Source: CAD feature listing. Evaluate the final solid. Frame: model axes, mm. A direction names the side the tool comes from. Give positions to 0.01 mm unless a question says otherwise; leave off trailing zeros. Order: outer loops, then holes, each group sorted by start corner. A loop starts at its lowest first (then second) coordinate and runs counter-clockwise, first axis right, second up.
```python
from build123d import *

# Parameters (mm, degrees)
EXTRUDE1_DEPTH           = 311.15
SKETCH2_R                = 5.207
SKETCH2_R_2              = 3.556
SKETCH2_R_3              = 6.731
CUT_WEB_HOLES_DEPTH      = 329.182750394
SKETCH3_R                = 6.731
SKETCH3_R_2              = 5.207
CUT_FLG_HOLES_DEPTH      = 329.182750394
CUT_FLG_HOLES_DEPTH_BACK = 329.182750394
SKETCH6_R                = 5.207
VLV_MODULATOR_DEPTH      = 329.182750394


with BuildPart() as part:
    # Sketch1 → Extrude1 (new, symmetric)
    with BuildSketch(Plane(origin=(0, 0, 0), x_dir=(0, 0, -1), z_dir=(1, 0, 0))):
        with BuildLine():
            Line((57.15, 87.3125), (12.7, 87.3125))
            ThreePointArc((12.7, 87.3125), (3.719743879, 83.592756121), (0, 74.6125))
            Line((0, 74.6125), (0, -74.6125))
            ThreePointArc((0, -74.6125), (3.719743879, -83.592756121), (12.7, -87.3125))
            Line((12.7, -87.3125), (57.15, -87.3125))
            Line((57.15, -87.3125), (57.15, -80.9625))
            Line((57.15, -80.9625), (12.7, -80.9625))
            ThreePointArc((12.7, -80.9625), (8.209871939, -79.102628061), (6.35, -74.6125))
            Line((6.35, -74.6125), (6.35, 74.6125))
            ThreePointArc((6.35, 74.6125), (8.209871939, 79.102628061), (12.7, 80.9625))
            Line((12.7, 80.9625), (57.15, 80.9625))
            Line((57.15, 80.9625), (57.15, 87.3125))
        make_face()
    extrude(amount=EXTRUDE1_DEPTH, both=True)

    # Sketch2 → Cut-Web Holes (cut, through all)
    with BuildSketch(Plane.XY):
        with Locations((-185.7375, 52.3875)):
            Circle(SKETCH2_R)
        with Locations((-261.9375, -4.7625)):
            Circle(SKETCH2_R_2)
        with Locations((-288.925, -42.8625)):
            Circle(SKETCH2_R_2)
        with Locations((-152.4, -42.8625)):
            Circle(SKETCH2_R)
        with Locations((-127, -30.1625)):
            Circle(SKETCH2_R_3)
        with Locations((-127, 33.3375)):
            Circle(SKETCH2_R_3)
        with Locations((-98.425, 52.3875)):
            Circle(SKETCH2_R)
        with Locations((-58.7375, 12.7)):
            Circle(SKETCH2_R)
        with Locations((-58.7375, -36.5125)):
            Circle(SKETCH2_R_3)
        with Locations((-185.7375, 1.5875)):
            Circle(SKETCH2_R)
        with Locations((-147.6375, 39.6875)):
            Circle(SKETCH2_R_2)
        with Locations((147.6375, 39.6875)):
            Circle(SKETCH2_R_2)
        with Locations((98.425, 52.3875)):
            Circle(SKETCH2_R)
        with Locations((127, 33.3375)):
            Circle(SKETCH2_R_3)
        with Locations((185.7375, 52.3875)):
            Circle(SKETCH2_R)
        with Locations((185.7375, 1.5875)):
            Circle(SKETCH2_R)
        with Locations((261.9375, -4.7625)):
            Circle(SKETCH2_R_2)
        with Locations((288.925, -42.8625)):
            Circle(SKETCH2_R_2)
        with Locations((152.4, -42.8625)):
            Circle(SKETCH2_R)
        with Locations((127, -30.1625)):
            Circle(SKETCH2_R_3)
        with Locations((58.7375, 12.7)):
            Circle(SKETCH2_R)
        with Locations((58.7375, -36.5125)):
            Circle(SKETCH2_R_3)
    extrude(amount=-CUT_WEB_HOLES_DEPTH, mode=Mode.SUBTRACT)

    # Sketch3 → Cut-Flg Holes (cut, two sides)
    with BuildSketch(Plane(origin=(0, 0, 0), x_dir=(1, 0, 0), z_dir=(0, 1, 0))) as cut_flg_holes_sk:
        with Locations(Location((-285.75, 38.1, 0), (0, 0, 270))):
            Circle(SKETCH3_R)
        with Locations(Location((-215.9, 38.1, 0), (0, 0, 270))):
            Circle(SKETCH3_R)
        with Locations(Location((285.75, 38.1, 0), (0, 0, 90))):
            Circle(SKETCH3_R)
        with Locations(Location((215.9, 38.1, 0), (0, 0, 90))):
            Circle(SKETCH3_R)
        with Locations(Location((165.1, 38.1, 0), (0, 0, 270))):
            Circle(SKETCH3_R)
        with Locations(Location((31.75, 38.1, 0), (0, 0, 270))):
            Circle(SKETCH3_R_2)
        with Locations(Location((-31.75, 38.1, 0), (0, 0, 270))):
            Circle(SKETCH3_R_2)
        with Locations(Location((-165.1, 38.1, 0), (0, 0, 270))):
            Circle(SKETCH3_R)
    extrude(amount=CUT_FLG_HOLES_DEPTH, mode=Mode.SUBTRACT)
    extrude(cut_flg_holes_sk.sketch, amount=-CUT_FLG_HOLES_DEPTH_BACK, mode=Mode.SUBTRACT)

    # Sketch6 → VLV-MODULATOR (cut, through all)
    with BuildSketch(Plane.XY):
        with Locations((-152.4, 52.3875)):
            Circle(SKETCH6_R)
        with Locations((-223.8375, 31.75)):
            Circle(SKETCH6_R)
        with Locations((-152.4, 22.225)):
            Circle(SKETCH6_R)
        with Locations((-223.8375, 1.5875)):
            Circle(SKETCH6_R)
        with Locations((223.8375, 1.5875)):
            Circle(SKETCH6_R)
        with Locations((152.4, 22.225)):
            Circle(SKETCH6_R)
        with Locations((152.4, 52.3875)):
            Circle(SKETCH6_R)
        with Locations((223.8375, 31.75)):
            Circle(SKETCH6_R)
    extrude(amount=-VLV_MODULATOR_DEPTH, mode=Mode.SUBTRACT)


solid = part.part
```
1) Draft query along Z for faces 1 (the cylindrical face through (-28.231, -84.093, -41.938)), 2 (the cylindrical face through (4.36, 83.69, -3.82)), 3 (the flat face through (311.15, 0, -5)). Return one class per face: +Z half, -Z half, draft (parallel to the pull), parting line (faces both ways), or undercut.
Report:
face 1: undercut
face 2: +Z half
face 3: draft
2) Section query B-B, the plane y = 63. Return the cut outline in (x, z).
Report:
outline: (-311.15, -6.35) - (311.15, -6.35) - (311.15, 0) - (-311.15, 0) - close
3) Reachability of faces 4 (the cylindrical face through (133.42, -28.14, -3.13)), 5 (the flat face through (4, -80.962, -35)) from +Z, -Z, +X, -X, +Y, -Y: full face, straight path, thin tool, end or side. Return the list, or none.
Report:
face 4: +Z, -Z
face 5: -Z, +X, -X
4) Section query A-A, the plane x = 127. Return the cut outline in (y, z).
Report:
outline: (-87.31, -57.15) - (-80.96, -57.15) - (-80.96, -12.7) arc R6.35 cw to (-74.61, -6.35) - (-36.89, -6.35) - (-36.89, 0) - (-74.61, 0) arc R12.7 ccw to (-87.31, -12.7) - close; (-23.43, -6.35) - (26.61, -6.35) - (26.61, 0) - (-23.43, 0) - close; (40.07, -6.35) - (74.61, -6.35) arc R6.35 cw to (80.96, -12.7) - (80.96, -57.15) - (87.31, -57.15) - (87.31, -12.7) arc R12.7 ccw to (74.61, 0) - (40.07, 0) - close
5) Material intervals for L1, parallel to Y at x = -271.5, z = -42; L2, parallel to Z at x = -105, y = -25, sorted ascending.
Report:
L1: y = -87.31 to -80.96, 80.96 to 87.31
L2: z = -6.35 to 0
6) Section query C-C, the plane x = -31.75. Return the cut outline in (y, z).
Report:
outline: (-87.31, -57.15) - (-80.96, -57.15) - (-80.96, -43.31) - (-87.31, -43.31) - close; (-87.31, -32.89) - (-80.96, -32.89) - (-80.96, -12.7) arc R6.35 cw to (-74.61, -6.35) - (74.61, -6.35) arc R6.35 cw to (80.96, -12.7) - (80.96, -32.89) - (87.31, -32.89) - (87.31, -12.7) arc R12.7 ccw to (74.61, 0) - (-74.61, 0) arc R12.7 ccw to (-87.31, -12.7) - close; (80.96, -57.15) - (87.31, -57.15) - (87.31, -43.31) - (80.96, -43.31) - close
7) Pin query (flat end, axial travel): pin 1 (12 mm diameter, centred on x = -185.74, y = 52.39, fed in from -Z). Return the tip coordinate at first contact, or that it passes through.
Report:
pin 1: stops at z = -6.35
